Source: three-view drawing plus pictorial views. Frame: mm from the lowest corner of the part. Round coordinates to 2 decimals unless told otherwise and drop trailing zeros. Loops run counter-clockwise (first coordinate to the right, second up) from the corner with the lowest first, then second, coordinate; pieces in that order, holes last. Notation, with made-up numbers: M 41,88 L 49,88 A16 ccw 49,113 Z; hole C 89.25,47 d10. An arc over 180 degrees is marked long. Answer as a JSON object with one key per item and string values.
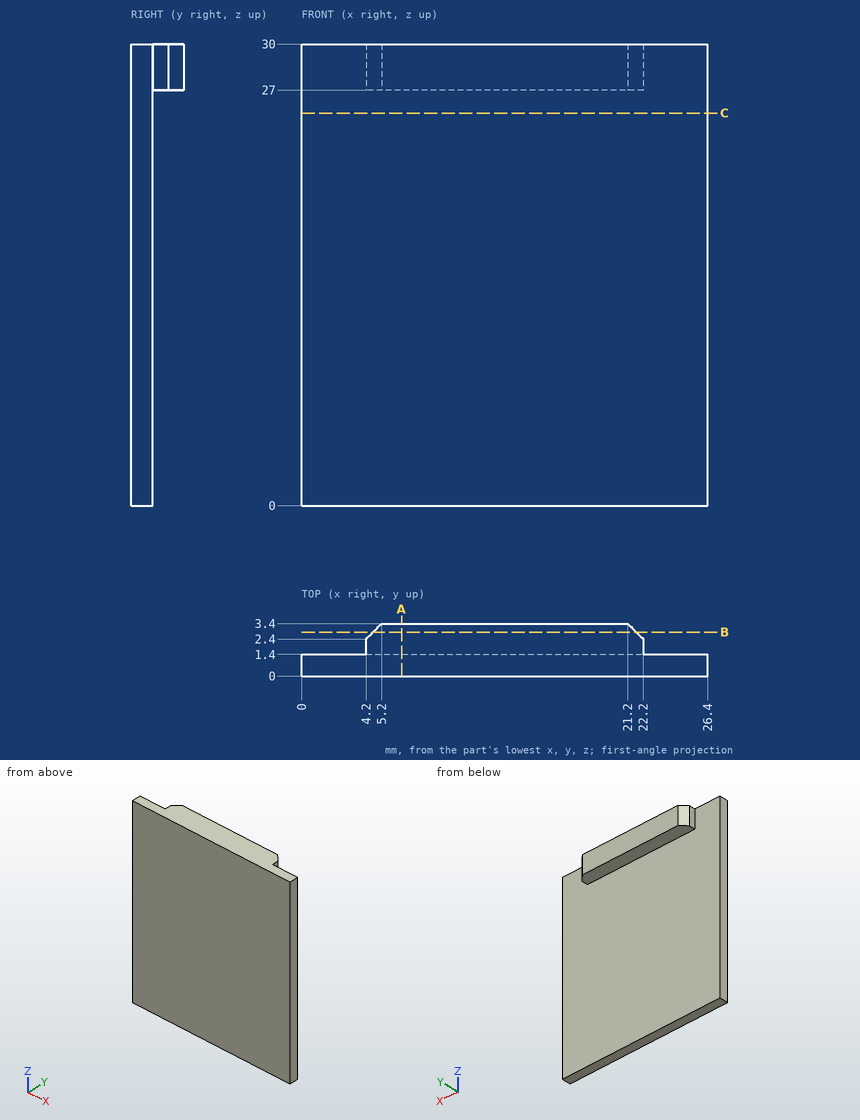
1) Cut plane C-C on z = 25.5. Return the cut outline in (x, y), and give its area (3 significant figures).
Geometry results:
{"outline": "M 0,0 L 26.4,0 L 26.4,1.4 L 0,1.4 Z", "area": "37.0 mm2"}
2) Cut plane A-A on x = 6.5. Return the cut outline in (y, z), and give its area (3 significant figures).
Geometry results:
{"outline": "M 0,0 L 1.4,0 L 1.4,27 L 3.4,27 L 3.4,30 L 0,30 Z", "area": "48.0 mm2"}
3) Line query: probe 1 along Y at (x, z) = (7.5, 24.75); probe 2 along Z at (x, y) = (8, 2.9). Output: solid intervals per line, ascending.
Geometry results:
{"probe 1": "0 to 1.4", "probe 2": "27 to 30"}
4) First-contact query: pin 1 (5 mm diameter, centred on x = 4.5, z = 5, fed in from +Y); pin 2 (1.1 mm diameter, centred on y = 2, z = 29, fed in from -X); pin 3 (1.5 mm diameter, centred on x = 20.5, y = 2.5, fed in from -Z). Flat tips, straight axial feed; report the tip coordinate or a pass-through.
Geometry results:
{"pin 1": "y = 1.4", "pin 2": "x = 4.2", "pin 3": "z = 27"}
5) Cut plane B-B on y = 2.85. Return the cut outline in (x, z).
Geometry results:
{"outline": "M 4.65,27 L 21.75,27 L 21.75,30 L 4.65,30 Z"}
